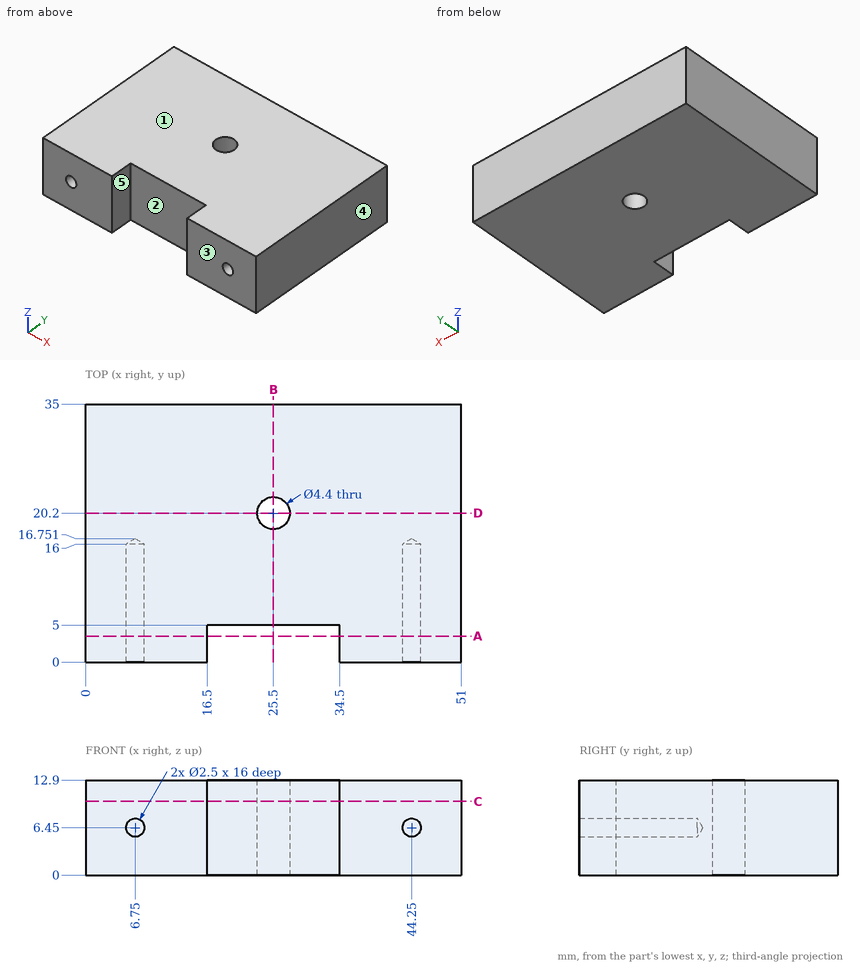
Part print with two shaded views. Sizes in mm from the minimum x, y, z corner. A direction names the side the tool comes from. Round coordinates to 2 decimals unless told otherwise and drop trailing zeros. Loops run counter-clockwise (first coordinate to the right, second up) from the corner with the lowest first, then second, coordinate; pieces in that order, holes last. Notation, with made-up numbers: (-13.75, 2.25) - (1.25, 2.25) arc R20 cw to (1.25, 33.25) - close; hole circle Ø2 at (3, 49.5). An arc over 180 degrees is marked (long way). Answer as a JSON object with one key per item and string values.
Item 1: Wall check: L1, parallel to X at y = 12.5, z = 6.45; L2, parallel to Y at x = 25.5, z = 3.25; L3, parallel to X at y = 3.5, z = 2.25. Give the ranges that are in metal, low to high.
Output:
{"L1": "0 to 5.5, 8 to 43, 45.5 to 51", "L2": "5 to 18, 22.4 to 35", "L3": "0 to 16.5, 34.5 to 51"}
Item 2: Pull direction X, two halves, no side cores. Call the marked faces 3, 4 and 5: pulls with the +X half, pulls with the -X half, needs draft (parallel to the pull), parting line crosses it, or undercut.
Output:
{"face 3": "needs draft", "face 4": "pulls with the +X half", "face 5": "undercut"}
Item 3: Band-saw the part on A-A on y = 3.5. List the corners of the cut face in (x, z), plus the area to 3 significant figures.
Output:
{"outline": "(0, 0) - (16.5, 0) - (16.5, 12.9) - (0, 12.9) - close; (34.5, 0) - (51, 0) - (51, 12.9) - (34.5, 12.9) - close; hole circle Ø2.5 at (6.75, 6.45); hole circle Ø2.5 at (44.25, 6.45)", "area": "416 mm2"}
Item 4: Band-saw the part on C-C on z = 10. List the corners of the cut face in (x, y).
Output:
{"outline": "(0, 0) - (16.5, 0) - (16.5, 5) - (34.5, 5) - (34.5, 0) - (51, 0) - (51, 35) - (0, 35) - close; hole circle Ø4.4 at (25.5, 20.2)"}
Item 5: Tool access for the marked faces 1 and 2: list every direction of +Z, -Z, +X, -X, +Y, -Y with a clear straight run to the whole face (end or side of a thin tool).
Output:
{"face 1": "+Z, +X, -X, +Y, -Y", "face 2": "+Z, -Z, -Y"}
Item 6: Band-saw the part on D-D on y = 20.2. List the corners of the cut face in (x, z).
Output:
{"outline": "(0, 0) - (23.3, 0) - (23.3, 12.9) - (0, 12.9) - close; (27.7, 0) - (51, 0) - (51, 12.9) - (27.7, 12.9) - close"}
Item 7: Band-saw the part on B-B on x = 25.5. List the corners of the cut face in (y, z).
Output:
{"outline": "(5, 0) - (18, 0) - (18, 12.9) - (5, 12.9) - close; (22.4, 0) - (35, 0) - (35, 12.9) - (22.4, 12.9) - close"}
